For this review, take the finished solid that the model builds, in its own axes (mm). A direction names the side the tool comes from. Give positions to 0.01 mm unless a question says otherwise; leave off trailing zeros. Loops run counter-clockwise (first coordinate to the right, second up) from the corner with the lowest first, then second, coordinate; pieces in that order, holes last. Notation, with made-up numbers: (7, -35) - (26, -35) arc R27 cw to (26, -17) - close; hole circle Ø2 at (7, 50). An arc over 180 degrees is marked (long way). Put each result on its own line as item: value.
from build123d import *

# Parameters (mm, degrees)
SERIES_PLATE_21_6_X_8_5_X_0_5_SKETCH_W = 21.6
SERIES_PLATE_21_6_X_8_5_X_0_5_SKETCH_H = 0.5
SERIES_PLATE_21_6_X_8_5_X_0_5_DEPTH    = 8.5


with BuildPart() as part:
    # Series Plate 21.6 x 8.5 x 0.5 Sketch → Series Plate 21.6 x 8.5 x 0.5 (new body)
    with BuildSketch(Plane(origin=(0, 1.95, 0), x_dir=(1, 0, 0), z_dir=(0, 1, 0))):
        with Locations((20, 14.9)):
            Rectangle(SERIES_PLATE_21_6_X_8_5_X_0_5_SKETCH_W, SERIES_PLATE_21_6_X_8_5_X_0_5_SKETCH_H)
    extrude(amount=SERIES_PLATE_21_6_X_8_5_X_0_5_DEPTH)

    # Spring (compressed 4.3) Sketch → Spring (compressed 4.3) (revolve)
    with BuildSketch(Plane(origin=(0, 6.95, 0), x_dir=(1, 0, 0), z_dir=(0, 1, 0))):
        Polygon((16.8, 15.15), (17.3, 15.15), (16.3, 19.45), (15.8, 19.45), align=None)
    revolve(axis=Axis((14.3, 6.95, -14.15), (0, 0, -1)))

    # Dimple 0.9 Sketch → Dimple 0.9 (revolve)
    with BuildSketch(Plane(origin=(0, 6.95, 0), x_dir=(1, 0, 0), z_dir=(0, 1, 0))):
        with BuildLine():
            Line((25.7, 15.15), (28.2, 15.15))
            ThreePointArc((28.2, 15.15), (27.028533026, 15.818147293), (25.7, 16.05))
            Line((25.7, 16.05), (25.7, 15.15))
        make_face()
    revolve(axis=Axis((25.7, 6.95, -14.15), (0, 0, -1)))


solid = part.part
1) For faces 4 (the face through (14, 7, -15.15)), 5 (the face through (16, 7, -19.45)), list the 3-axis set-ups (+Z, -Z, +X, -X, +Y, -Y) from which the entire face can be reached by the end or side of a thin tool; tool diameter is ignored.
Geometry check:
face 4: none
face 5: -Z, +X, -X, +Y, -Y
2) Wall thickness on line 1 (Z direction, x = 19.5, y = 4.5); line 2 (X direction, y = 7.25, z = -18.5); line 3 (Y direction, x = 14.25, z = -17.7): over which ranges is each line inside the solid? List them lowest first.
Geometry check:
line 1: z = -15.15 to -14.65
line 2: x = 12.1 to 12.61, 15.99 to 16.5
line 3: y = 4.54 to 5.04, 8.86 to 9.36
3) Take a section at C-C on z = -18.25. State the section outline as (x, y) points, and give its area (3 significant figures).
Geometry check:
outline: circle Ø4.56 at (14.3, 6.95); hole circle Ø3.56 at (14.3, 6.95)
area: 6.37 mm²
4) Take a section at D-D on y = 3.5. State the section outline as (x, z) points.
Geometry check:
outline: (9.2, -15.15) - (30.8, -15.15) - (30.8, -14.65) - (9.2, -14.65) - close
5) Take a section at B-B on y = 6.95. State the section outline as (x, z) points, and give its area (3 significant figures).
Geometry check:
outline: (9.2, -15.15) - (11.3, -15.15) - (12.3, -19.45) - (12.8, -19.45) - (11.8, -15.15) - (16.8, -15.15) - (15.8, -19.45) - (16.3, -19.45) - (17.3, -15.15) - (23.2, -15.15) arc R3.92 ccw to (28.2, -15.15) - (30.8, -15.15) - (30.8, -14.65) - (9.2, -14.65) - close
area: 18.2 mm²
6) Insertion check: pin 1 Ø1.5 at (x, y) = (15, 7) entering from -Z; pin 2 Ø2 at (x, z) = (13.5, -18.5) entering from +Y. Each pin has a flat end and moves straight along its axis. Give the tip position at first contact, or say it passes through.
Geometry check:
pin 1: stops at z = -15.15
pin 2: stops at y = 9.35
7) Take a section at A-A on x = 14.3. State the section outline as (y, z) points, and give its area (3 significant figures).
Geometry check:
outline: (1.95, -15.15) - (3.95, -15.15) - (4.95, -19.45) - (5.45, -19.45) - (4.45, -15.15) - (9.45, -15.15) - (8.45, -19.45) - (8.95, -19.45) - (9.95, -15.15) - (10.45, -15.15) - (10.45, -14.65) - (1.95, -14.65) - close
area: 8.55 mm²
8) Draft analysis for pull direction Z (two halves, no side actions). For faces 1 (the face through (15.319, 5.351, -17.748)), 2 (the face through (16.57, 6.23, -17.81)), 3 (the face through (20, 6, -14.65)), state which applies: pulls with the +Z half, pulls with the -Z half, needs draft (parallel to the pull), parting line crosses it, or undercut.
Geometry check:
face 1: undercut
face 2: pulls with the -Z half
face 3: pulls with the +Z half
